Geometry: final body of the model. Coordinates: model frame, mm. Give positions to 0.01 mm unless a question says otherwise; leave off trailing zeros. Write each loop counter-clockwise with the first axis right and the second up, starting at its lowest first coordinate (ties: lowest second). Pieces come first, ordered by that corner, then holes. Notation, with made-up numbers: M 67,-22 L 85,-22 A12 ccw 85,-6 Z; hole C -14.75,83.25 d5. An arc over 180 degrees is marked long. Use a Markdown table: item, result. Add a question column.
(1) Cut plane D-D (x = 131). Output: boundary loops of the cut face in (y, z), plus the area to 4 significant figures.
(2) Pin query (flat end, axial travel): pin 1 Ø3 at (x, y) = (97, 73) entering from +Z; pin 2 Ø1.5 at (y, z) = (40, -4) entering from +X; pin 3 Ø2 at (y, z) = (62.5, -6.5) entering from +X. Return the tip coordinate at first contact, or that it passes through.
(3) Cut plane A-A (z = -3.25). State how many separate pieces and enclosed holes the cut face has, plus the area to 3 significant figures.
(4) Cut plane B-B (y = 31.5). Output: boundary loops of the cut face in (x, z).
(5) Cut plane C-C (x = 112). Output: boundary loops of the cut face in (y, z), plus the area to 4 significant figures.
(6) Material intervals for L1, parallel to Y at x = 170, z = -3.6; L2, parallel to Y at x = 72, z = -3.25; L3, parallel to Y at x = 136, z = -3, sorted ascending.
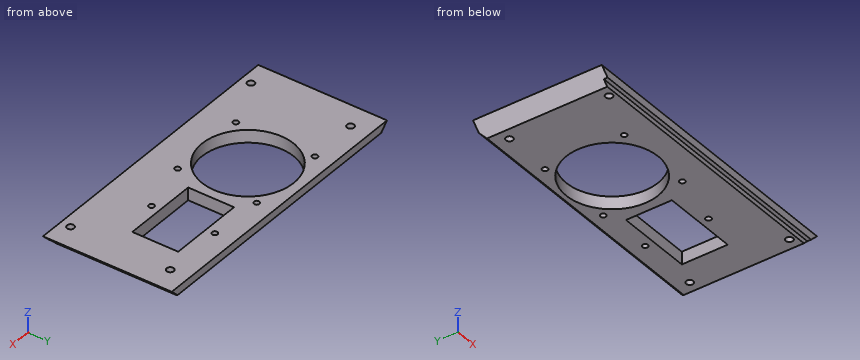
```python
from build123d import *

# Parameters (mm, degrees)
SKETCH1_W           = 185
SKETCH1_H           = 84
SKETCH1_R           = 2.25
BOSS_EXTRUDE1_DEPTH = 5
SKETCH2_W           = 185
SKETCH2_H           = 79
SKETCH2_R           = 2.25
BOSS_EXTRUDE2_DEPTH = 3
CHAMFER1_SIZE       = 8
CHAMFER3_SIZE       = 3
SKETCH3_W           = 7.071067812
SKETCH3_H           = 2.6
CUT_EXTRUDE1_DEPTH  = 221.270985121
SKETCH4_R           = 29
SKETCH4_R_2         = 1.75
SKETCH4_W           = 48
SKETCH4_H           = 29
CUT_EXTRUDE2_DEPTH  = 204.334699449


with BuildPart() as part:
    # Sketch1 → Boss-Extrude1 (new body)
    with BuildSketch(Plane.XY):
        with Locations((92.5, 42)):
            Rectangle(SKETCH1_W, SKETCH1_H)
        with Locations((15, 9)):
            Circle(SKETCH1_R, mode=Mode.SUBTRACT)
        with Locations(Location((170, 9, 0), (0, 0, 180))):
            Circle(SKETCH1_R, mode=Mode.SUBTRACT)
        with Locations((15, 72)):
            Circle(SKETCH1_R, mode=Mode.SUBTRACT)
        with Locations(Location((170, 72, 0), (0, 0, 180))):
            Circle(SKETCH1_R, mode=Mode.SUBTRACT)
    extrude(amount=-BOSS_EXTRUDE1_DEPTH)

    # Sketch2 → Boss-Extrude2 (add)
    with BuildSketch(Plane(origin=(0, 0, -5), x_dir=(-1, 0, 0), z_dir=(0, 0, -1))):
        with Locations((-92.5, 44.5)):
            Rectangle(SKETCH2_W, SKETCH2_H)
        with Locations(Location((-15, 9, 0), (0, 0, 180))):
            Circle(SKETCH2_R, mode=Mode.SUBTRACT)
        with Locations((-170, 9)):
            Circle(SKETCH2_R, mode=Mode.SUBTRACT)
        with Locations(Location((-15, 72, 0), (0, 0, 180))):
            Circle(SKETCH2_R, mode=Mode.SUBTRACT)
        with Locations((-170, 72)):
            Circle(SKETCH2_R, mode=Mode.SUBTRACT)
    extrude(amount=BOSS_EXTRUDE2_DEPTH)

    # Chamfer1
    # the kernel refuses this chamfer: 8 mm, written as the material it takes off along each edge
    with BuildSketch(Plane(origin=(185, -15.573463904, -8), x_dir=(-0.9996219169112968, 0, -0.027495876610586296), z_dir=(0, 1, 0)), Plane(origin=(0, 104.573463904, -8), x_dir=(0.9996219169112968, 0, -0.027495876610586275), z_dir=(0, -1, 0))) as chamfer1_piece_1:
        Polygon((CHAMFER1_SIZE * 0.999621916911, CHAMFER1_SIZE * 0.0274958766106), (-CHAMFER1_SIZE * 0.0274958766106, CHAMFER1_SIZE * 0.999621916911), (0, 0), align=None)
    extrude(amount=120.146927807, mode=Mode.SUBTRACT)

    # Chamfer3
    chamfer3_edges = [part.edges().sort_by_distance(p)[0] for p in [
        (92.5, 84, -8),
    ]]
    chamfer(chamfer3_edges, length=CHAMFER3_SIZE)

    # Sketch3 → Cut-Extrude1 (cut, through all, along a direction that is not the sketch's normal)
    with BuildSketch(Plane(origin=(92.5, 0, -92.5), x_dir=(-0.7071067811865452, 0, -0.7071067811865498), z_dir=(0.7071067811865498, 0, -0.7071067811865452))):
        with Locations((-127.279220614, 1.3)):
            Rectangle(SKETCH3_W, SKETCH3_H)
    extrude(amount=-CUT_EXTRUDE1_DEPTH, dir=(1, 0, 0), mode=Mode.SUBTRACT)

    # Sketch4 → Cut-Extrude2 (cut, through all)
    with BuildSketch(Plane.XY):
        with Locations((72, 49)):
            Circle(SKETCH4_R)
        with Locations((47, 73)):
            Circle(SKETCH4_R_2)
        with Locations((97, 73)):
            Circle(SKETCH4_R_2)
        with Locations((97, 23)):
            Circle(SKETCH4_R_2)
        with Locations((47, 23)):
            Circle(SKETCH4_R_2)
        with Locations((131, 71.5)):
            Circle(SKETCH4_R_2)
        with Locations((131, 31.5)):
            Circle(SKETCH4_R_2)
        with Locations((131, 51.5)):
            Rectangle(SKETCH4_W, SKETCH4_H)
    extrude(amount=-CUT_EXTRUDE2_DEPTH, mode=Mode.SUBTRACT)


solid = part.part
```
Answer list:
| question | item | result |
|---|---|---|
| 1 | outline | M 2.6,-5 L 5,-5 L 5,-8 L 29.75,-8 L 29.75,0 L 2.6,0 Z; M 33.25,-8 L 37,-8 L 37,0 L 33.25,0 Z; M 66,-8 L 69.75,-8 L 69.75,0 L 66,0 Z; M 73.25,-8 L 81,-8 L 84,-5 L 84,0 L 73.25,0 Z |
| 1 | area | 351.5 mm² |
| 2 | pin 1 | through |
| 2 | pin 2 | x = 181.75 |
| 2 | pin 3 | x = 179.5 |
| 3 | separate pieces | 1 |
| 3 | enclosed holes | 12 |
| 3 | area | 10,400 mm² |
| 4 | outline | M 0,0 L 8,-8 L 48.88,-8 L 48.88,0 Z; M 95.12,-8 L 129.25,-8 L 129.25,0 L 95.12,0 Z; M 132.75,-8 L 177,-8 L 185,0 L 132.75,0 Z |
| 5 | outline | M 2.6,-5 L 5,-5 L 5,-8 L 37,-8 L 37,0 L 2.6,0 Z; M 66,-8 L 81,-8 L 84,-5 L 84,0 L 66,0 Z |
| 5 | area | 407.5 mm² |
| 6 | L1 | 2.6 to 6.75, 11.25 to 69.75, 74.25 to 84 |
| 6 | L2 | 2.6 to 20, 78 to 84 |
| 6 | L3 | 2.6 to 37, 66 to 84 |
